CAD build for the part. Positions are in the model's coordinates, mm. Face numbers are marked on the shaded views. A direction names the side the tool comes from. Round coordinates to 2 decimals unless told otherwise and drop trailing zeros. Order: outer loops, then holes, each group sorted by start corner. A loop starts at its lowest first (then second) coordinate and runs counter-clockwise, first axis right, second up. Notation, with made-up numbers: (64.25, -29) - (104.25, -29) arc R8 cw to (104.25, -14) - close; hole circle Ø4 at (70.25, 31.25). An arc over 180 degrees is marked (long way). Write item = value, one per line.
from build123d import *

# Parameters (mm, degrees)
BOSS_EXTRUDE3_DEPTH = 4
BOSS_EXTRUDE4_START = -15
BOSS_EXTRUDE4_DEPTH = 15
SKETCH3_R           = 2.75
CUT_EXTRUDE1_DEPTH  = 74


with BuildPart() as part:
    # Sketch2 → Boss-Extrude3 (new body)
    with BuildSketch(Plane(origin=(0, 0, 0), x_dir=(1, 0, 0), z_dir=(0, 1, 0))):
        with BuildLine():
            Line((45, 20), (-27.5, 20))
            Line((-27.5, 20), (-27.5, 0))
            Line((-27.5, 0), (-8.1, 0))
            ThreePointArc((-8.1, 0), (0, 8.1), (8.1, 0))
            Line((8.1, 0), (36.9, 0))
            ThreePointArc((36.9, 0), (39.272435072, 5.727564928), (45, 8.1))
            Line((45, 8.1), (45, 20))
        make_face()
        with BuildLine():
            ThreePointArc((8.1, 0), (0, 8.1), (-8.1, 0))
            Line((-8.1, 0), (-6.6, 0))
            ThreePointArc((-6.6, 0), (0, 6.6), (6.6, 0))
            Line((6.6, 0), (8.1, 0))
        make_face()
        with BuildLine():
            Line((-6.6, 0), (-8.1, 0))
            ThreePointArc((-8.1, 0), (0, -8.1), (8.1, 0))
            Line((8.1, 0), (6.6, 0))
            ThreePointArc((6.6, 0), (0, -6.6), (-6.6, 0))
        make_face()
        with BuildLine():
            ThreePointArc((53.1, 0), (50.727564928, 5.727564928), (45, 8.1))
            Line((45, 8.1), (45, 6.6))
            ThreePointArc((45, 6.6), (49.666904756, 4.666904756), (51.6, 0))
            Line((51.6, 0), (53.1, 0))
        make_face()
        with BuildLine():
            Line((45, 6.6), (45, 8.1))
            ThreePointArc((45, 8.1), (39.272435072, 5.727564928), (36.9, 0))
            Line((36.9, 0), (38.4, 0))
            ThreePointArc((38.4, 0), (40.333095244, 4.666904756), (45, 6.6))
        make_face()
        with BuildLine():
            ThreePointArc((36.9, 0), (45, -8.1), (53.1, 0))
            Line((53.1, 0), (51.6, 0))
            ThreePointArc((51.6, 0), (45, -6.6), (38.4, 0))
            Line((38.4, 0), (36.9, 0))
        make_face()
        with BuildLine():
            ThreePointArc((81.9, 0), (90, -8.1), (98.1, 0))
            Line((98.1, 0), (96.6, 0))
            ThreePointArc((96.6, 0), (90, -6.6), (83.4, 0))
            Line((83.4, 0), (81.9, 0))
        make_face()
        with BuildLine():
            Line((96.6, 0), (98.1, 0))
            ThreePointArc((98.1, 0), (90, 8.1), (81.9, 0))
            Line((81.9, 0), (83.4, 0))
            ThreePointArc((83.4, 0), (90, 6.6), (96.6, 0))
        make_face()
        with BuildLine():
            Line((117.5, 20), (45, 20))
            Line((45, 20), (45, 8.1))
            ThreePointArc((45, 8.1), (50.727564928, 5.727564928), (53.1, 0))
            Line((53.1, 0), (81.9, 0))
            ThreePointArc((81.9, 0), (90, 8.1), (98.1, 0))
            Line((98.1, 0), (117.5, 0))
            Line((117.5, 0), (117.5, 20))
        make_face()
        with BuildLine():
            Line((-8.1, 0), (-27.5, 0))
            Line((-27.5, 0), (-27.5, -20))
            Line((-27.5, -20), (117.5, -20))
            Line((117.5, -20), (117.5, 0))
            Line((117.5, 0), (98.1, 0))
            ThreePointArc((98.1, 0), (90, -8.1), (81.9, 0))
            Line((81.9, 0), (53.1, 0))
            ThreePointArc((53.1, 0), (45, -8.1), (36.9, 0))
            Line((36.9, 0), (8.1, 0))
            ThreePointArc((8.1, 0), (0, -8.1), (-8.1, 0))
        make_face()
    extrude(amount=BOSS_EXTRUDE3_DEPTH)

    # Sketch2<5> → Boss-Extrude4 (add)
    with BuildSketch(Plane(origin=(0, 0, 0), x_dir=(1, 0, 0), z_dir=(0, 1, 0)).offset(BOSS_EXTRUDE4_START)):
        with BuildLine():
            ThreePointArc((8.1, 0), (0, 8.1), (-8.1, 0))
            Line((-8.1, 0), (-6.6, 0))
            ThreePointArc((-6.6, 0), (0, 6.6), (6.6, 0))
            Line((6.6, 0), (8.1, 0))
        make_face()
        with BuildLine():
            Line((-6.6, 0), (-8.1, 0))
            ThreePointArc((-8.1, 0), (0, -8.1), (8.1, 0))
            Line((8.1, 0), (6.6, 0))
            ThreePointArc((6.6, 0), (0, -6.6), (-6.6, 0))
        make_face()
        with BuildLine():
            ThreePointArc((53.1, 0), (50.727564928, 5.727564928), (45, 8.1))
            Line((45, 8.1), (45, 6.6))
            ThreePointArc((45, 6.6), (49.666904756, 4.666904756), (51.6, 0))
            Line((51.6, 0), (53.1, 0))
        make_face()
        with BuildLine():
            Line((45, 6.6), (45, 8.1))
            ThreePointArc((45, 8.1), (39.272435072, 5.727564928), (36.9, 0))
            Line((36.9, 0), (38.4, 0))
            ThreePointArc((38.4, 0), (40.333095244, 4.666904756), (45, 6.6))
        make_face()
        with BuildLine():
            ThreePointArc((36.9, 0), (45, -8.1), (53.1, 0))
            Line((53.1, 0), (51.6, 0))
            ThreePointArc((51.6, 0), (45, -6.6), (38.4, 0))
            Line((38.4, 0), (36.9, 0))
        make_face()
        with BuildLine():
            ThreePointArc((81.9, 0), (90, -8.1), (98.1, 0))
            Line((98.1, 0), (96.6, 0))
            ThreePointArc((96.6, 0), (90, -6.6), (83.4, 0))
            Line((83.4, 0), (81.9, 0))
        make_face()
        with BuildLine():
            Line((96.6, 0), (98.1, 0))
            ThreePointArc((98.1, 0), (90, 8.1), (81.9, 0))
            Line((81.9, 0), (83.4, 0))
            ThreePointArc((83.4, 0), (90, 6.6), (96.6, 0))
        make_face()
    extrude(amount=BOSS_EXTRUDE4_DEPTH)

    # Sketch3 → Cut-Extrude1 (cut)
    with BuildSketch(Plane.XZ):
        with BuildLine():
            ThreePointArc((19.75, 0), (22.5, -2.75), (25.25, 0))
            Line((25.25, 0), (19.75, 0))
        make_face()
        with BuildLine():
            Line((19.75, 0), (25.25, 0))
            ThreePointArc((25.25, 0), (22.5, 2.75), (19.75, 0))
        make_face()
        with Locations(Location((67.5, 0, 0), (0, 0, 270))):
            Circle(SKETCH3_R)
    extrude(amount=-CUT_EXTRUDE1_DEPTH, mode=Mode.SUBTRACT)


solid = part.part
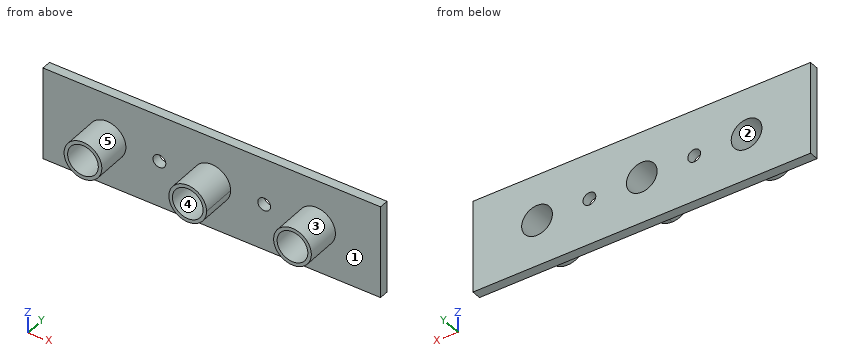
(1) Pull direction Z, two halves, no side cores. Call the marked faces 1, 2 and 3: released by +Z, released by -Z, zero draft, split by the parting line, or undercut.
Solved:
face_1 = zero draft
face_2 = undercut
face_3 = split by the parting line
(2) Band-saw the part on D-D on z = 9.5. List the corners of the cut face in (x, y).
Solved:
outline = (-27.5, 0) - (117.5, 0) - (117.5, 4) - (-27.5, 4) - close
(3) Band-saw the part on C-C on x = 0. List the corners of the cut face in (y, z), plus the area to 3 significant figures.
Solved:
outline = (-15, -8.1) - (0, -8.1) - (0, -20) - (4, -20) - (4, -6.6) - (-15, -6.6) - close; (-15, 6.6) - (4, 6.6) - (4, 20) - (0, 20) - (0, 8.1) - (-15, 8.1) - close
area = 152 mm²
(4) Probe line 1 along X through (y, z) = (-0.5, -1.5); line 2 along Z through (x, y) = (90, -1.25); line 3 along Y through (x, z) = (99.5, 10). List the from-to ranges inside material, lowest first.
Solved:
line_1 = -7.96 to -6.43, 6.43 to 7.96, 37.04 to 38.57, 51.43 to 52.96, 82.04 to 83.57, 96.43 to 97.96
line_2 = -8.1 to -6.6, 6.6 to 8.1
line_3 = 0 to 4
(5) Band-saw the part on A-A on y = -6.5. List the corners of the cut face in (x, z).
Solved:
outline = circle Ø16.2 at (0, 0); circle Ø16.2 at (45, 0); circle Ø16.2 at (90, 0); hole circle Ø13.2 at (0, 0); hole circle Ø13.2 at (45, 0); hole circle Ø13.2 at (90, 0)
(6) Band-saw the part on B-B on x = 67.5. List the corners of the cut face in (y, z), plus the area to 3 significant figures.
Solved:
outline = (0, -20) - (4, -20) - (4, -2.75) - (0, -2.75) - close; (0, 2.75) - (4, 2.75) - (4, 20) - (0, 20) - close
area = 138 mm²
(7) Drop flat-ended pins along their axis: pin 1 (1.5 mm diameter, centred on x = 51, z = -15, fed in from -Y); pin 2 (3 mm diameter, centred on x = 95.5, y = -11, fed in from -Z); pin 3 (8 mm diameter, centred on x = 42, y = -8, fed in from +Z). Give the stop position or say it passes through.
Solved:
pin_1 = 0
pin_2 = -7.04
pin_3 = 8.1
(8) Tool access for the marked faces 4 and 5: list every direction of +Z, -Z, +X, -X, +Y, -Y with a clear straight run to the whole face (end or side of a thin tool).
Solved:
face_4 = +Y, -Y
face_5 = -Y
